Input: part model. Units: mm. Frame: model coordinates. Face numbers are marked on the shaded views. Round coordinates to 2 decimals unless told otherwise and drop trailing zeros. Loops run counter-clockwise (first coordinate to the right, second up) from the corner with the lowest first, then second, coordinate; pieces in that order, holes last. Notation, with made-up numbers: (4, -34) -> (43, -34) arc R17 cw to (43, -30) -> close; hole circle Ø5 at (57, -4.75). An arc over 180 degrees is marked (long way). Answer as a JSON object with one key per item and string values.
```python
from build123d import *

# Parameters (mm, degrees)
F0_W     = 63.5
F0_H     = 63.5
F1_DEPTH = 6.35
F2_W     = 21.825
F2_H     = 6.35
F2_W_2   = 6.35
F2_H_2   = 21.825
F3_DEPTH = 3.81


with BuildPart() as f1:
    # F0 (on Top) → F1 (new body)
    with BuildSketch(Plane.XY):
        Rectangle(F0_W, F0_H)
    extrude(amount=F1_DEPTH)

    # F2 (on face) → F3 (cut)
    with BuildSketch(Plane.XY.offset(6.35)):
        with Locations((14.0875, 3.175)):
            Rectangle(F2_W, F2_H)
        with Locations((0, -10.9125)):
            Rectangle(F2_W_2, F2_H_2)
        with Locations((0, 3.175)):
            Rectangle(F2_W_2, F2_H)
        with Locations((-14.0875, 3.175)):
            Rectangle(F2_W, F2_H)
        with Locations((0, 17.2625)):
            Rectangle(F2_W_2, F2_H_2)
    extrude(amount=-F3_DEPTH, mode=Mode.SUBTRACT)


solid = f1.part
```
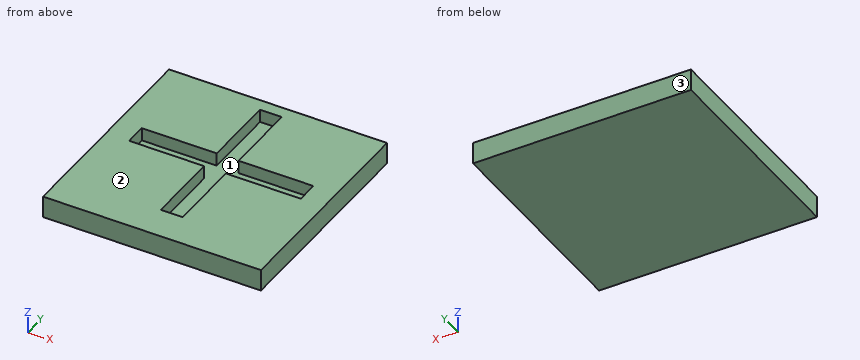
1) Section C-C, the plane x = 20. Output: boundary loops of the cut face in (y, z), plus the area to 3 significant figures.
Output:
{"outline": "(-31.75, 0) -> (31.75, 0) -> (31.75, 6.35) -> (6.35, 6.35) -> (6.35, 2.54) -> (0, 2.54) -> (0, 6.35) -> (-31.75, 6.35) -> close", "area": "379 mm^2"}
2) Ray query, probe 1 along Y at (x, z) = (12, 3.75); probe 2 along X at (y, z) = (10.5, 6.25) (3 decimals); probe 3 along X at (y, z) = (2, 3.5). Return the intervals inside material, ascending.
Output:
{"probe 1": "y = -31.75 to 0, 6.35 to 31.75", "probe 2": "x = -31.75 to -3.175, 3.175 to 31.75", "probe 3": "x = -31.75 to -25, 25 to 31.75"}
3) Section B-B, the plane z = 4. Output: boundary loops of the cut face in (x, y) (3 decimals).
Output:
{"outline": "(-31.75, -31.75) -> (31.75, -31.75) -> (31.75, 31.75) -> (-31.75, 31.75) -> close; hole (-25, 0) -> (-3.175, 0) -> (-3.175, -21.825) -> (3.175, -21.825) -> (3.175, 0) -> (25, 0) -> (25, 6.35) -> (3.175, 6.35) -> (3.175, 28.175) -> (-3.175, 28.175) -> (-3.175, 6.35) -> (-25, 6.35) -> close"}
4) Section A-A, the plane y = 12.5. Output: boundary loops of the cut face in (x, z) (3 decimals).
Output:
{"outline": "(-31.75, 0) -> (31.75, 0) -> (31.75, 6.35) -> (3.175, 6.35) -> (3.175, 2.54) -> (-3.175, 2.54) -> (-3.175, 6.35) -> (-31.75, 6.35) -> close"}
5) Draft query along Y for the marked faces 1, 2 and 3. Return one class per face: +Y half, -Y half, draft (parallel to the pull), parting line (faces both ways), or undercut.
Output:
{"face 1": "undercut", "face 2": "draft", "face 3": "+Y half"}
